Could you check a few things on this model? Use its own coordinates, in mm. A direction names the side the tool comes from. Give positions to 0.01 mm unless a question says otherwise; leave off trailing zeros. Loops run counter-clockwise (first coordinate to the right, second up) from the corner with the lowest first, then second, coordinate; pieces in that order, holes last. Notation, with made-up numbers: (-34, -33) -> (-1, -33) arc R12 cw to (-1, -26) -> close; hole circle Ø9 at (71.25, 62.5). An arc over 180 degrees is marked (long way). Write each question's results on one line, items separated by ' | '. Start each with the question number.
Q1. If we section it at C-C, the plane x = 32: List the corners of the cut face in (y, z) for me, plus the area to 3 significant figures.
Q2. If we section it at B-B, the plane y = -31: List the corners of the cut face in (x, z) for me, plus the area to 3 significant figures.
Q3. We'd pull the mould along X, two halves only. Please class faces 1 (the face through (-10, 69, 49)), 2 (the face through (13.17, 20.66, 104.93)), 3 (the face through (21, -21, 100)): released by +X, released by -X, zero draft, split by the parting line, or undercut.
Q4. Will these pins go through, and if not, where does the flat tip stop? P1, Ø1.5, axis at y = 43.5, z = 45.5, coming from the +X side; P2, Ø8, axis at x = -66, y = 67, coming from the +Z side; P3, Ø12, axis at y = 74.5, z = 53.5, coming from the +X side.
Q5. If I drill on line 1 along X through (y, z) = (12.5, 36); line 2 along X through (y, z) = (-16, 43); line 3 along Y through (x, z) = (21, 85), over which ranges is the centre line in solid material (lowest first)?
Q6. Which directions (+Z, -Z, +X, -X, +Y, -Y) give clear straight access to the entire face, cutting with the end or side of a thin tool? Please do faces 4 (the face through (21, -21, 0)), 5 (the face through (-64.237, 63.036, 49.3)), 6 (the face through (0, 0, -10)).
Q7. If we section it at A-A, the plane z = 63.5: List the corners of the cut face in (x, y) for me.
Q8. If we section it at D-D, the plane x = 0: List the corners of the cut face in (y, z) for me.
from build123d import *

# Parameters (mm, degrees)
SKETCH1_R                = 100
BOSS_EXTRUDE1_DEPTH      = 100
BOSS_EXTRUDE2_DEPTH      = 10
BOSS_EXTRUDE2_DEPTH_BACK = 110
SKETCH2_R                = 24.5


with BuildPart() as part:
    # Sketch1 → Boss-Extrude1 (new body)
    with BuildSketch(Plane.XY):
        Circle(SKETCH1_R)
        with BuildLine():
            Line((-10, 89.4427191), (-10, 48.989794856))
            ThreePointArc((-10, 48.989794856), (-35.355339059, 35.355339059), (-48.989794856, 10))
            Line((-48.989794856, 10), (-89.4427191, 10))
            ThreePointArc((-89.4427191, 10), (-63.639610307, 63.639610307), (-10, 89.4427191))
        make_face(mode=Mode.SUBTRACT)
        with BuildLine():
            Line((10, 89.4427191), (10, 48.989794856))
            ThreePointArc((10, 48.989794856), (35.355339059, 35.355339059), (48.989794856, 10))
            Line((48.989794856, 10), (89.4427191, 10))
            ThreePointArc((89.4427191, 10), (63.639610307, 63.639610307), (10, 89.4427191))
        make_face(mode=Mode.SUBTRACT)
        with BuildLine():
            Line((89.4427191, -10), (48.989794856, -10))
            ThreePointArc((48.989794856, -10), (35.355339059, -35.355339059), (10, -48.989794856))
            Line((10, -48.989794856), (10, -89.4427191))
            ThreePointArc((10, -89.4427191), (63.639610307, -63.639610307), (89.4427191, -10))
        make_face(mode=Mode.SUBTRACT)
        with BuildLine():
            Line((-10, -89.4427191), (-10, -48.989794856))
            ThreePointArc((-10, -48.989794856), (-35.355339059, -35.355339059), (-48.989794856, -10))
            Line((-48.989794856, -10), (-89.4427191, -10))
            ThreePointArc((-89.4427191, -10), (-63.639610307, -63.639610307), (-10, -89.4427191))
        make_face(mode=Mode.SUBTRACT)
    extrude(amount=BOSS_EXTRUDE1_DEPTH)

    # Sketch2 → Boss-Extrude2 (add, two sides: drawn at the far end of the back side and taken through both)
    with BuildSketch(Plane.XY.offset(100).offset(-BOSS_EXTRUDE2_DEPTH_BACK)):
        Circle(SKETCH2_R)
    extrude(amount=BOSS_EXTRUDE2_DEPTH + BOSS_EXTRUDE2_DEPTH_BACK)


solid = part.part
Final values:
1) outline: (-94.74, 0) -> (-84.12, 0) -> (-84.12, 100) -> (-94.74, 100) -> close; (-38.42, 0) -> (38.42, 0) -> (38.42, 100) -> (-38.42, 100) -> close; (84.12, 0) -> (94.74, 0) -> (94.74, 100) -> (84.12, 100) -> close | area: 9,810 mm²
2) outline: (-95.07, 0) -> (-84.49, 0) -> (-84.49, 100) -> (-95.07, 100) -> close; (-39.23, 0) -> (39.23, 0) -> (39.23, 100) -> (-39.23, 100) -> close; (84.49, 0) -> (95.07, 0) -> (95.07, 100) -> (84.49, 100) -> close | area: 9,960 mm²
3) face 1: undercut | face 2: split by the parting line | face 3: zero draft
4) P1: stops at x = 90.4 | P2: stops at z = 100 | P3: stops at x = 72.85
5) line 1: x = -99.22 to -89.13, -48.41 to 48.41, 89.13 to 99.22 | line 2: x = -98.71 to -88.57, -47.37 to 47.37, 88.57 to 98.71 | line 3: y = -97.77 to -87.52, -45.38 to 45.38, 87.52 to 97.77
6) face 4: -Z | face 5: +Z, -Z | face 6: -Z, +X, -X, +Y, -Y
7) outline: circle Ø200 at (0, 0); hole (-89.44, -10) arc R90 ccw to (-10, -89.44) -> (-10, -48.99) arc R50 cw to (-48.99, -10) -> close; hole (-89.44, 10) -> (-48.99, 10) arc R50 cw to (-10, 48.99) -> (-10, 89.44) arc R90 ccw to start; hole (10, -89.44) arc R90 ccw to (89.44, -10) -> (48.99, -10) arc R50 cw to (10, -48.99) -> close; hole (10, 48.99) arc R50 cw to (48.99, 10) -> (89.44, 10) arc R90 ccw to (10, 89.44) -> close
8) outline: (-100, 0) -> (-24.5, 0) -> (-24.5, -10) -> (24.5, -10) -> (24.5, 0) -> (100, 0) -> (100, 100) -> (24.5, 100) -> (24.5, 110) -> (-24.5, 110) -> (-24.5, 100) -> (-100, 100) -> close
